```python
from build123d import *

# Parameters (mm, degrees)
SKETCH1_W            = 64.75
SKETCH1_H            = 20
BODY_DEPTH           = 140
SHELL1_T             = 3
SWITCH_CUTOUT_REACH  = 148.722
SKETCH2_W            = 26.75
SKETCH2_H            = 12
SKETCH4_W            = 15
SKETCH4_H            = 27
SKETCH4_R            = 4.0125
AXLE_HOLDER_DEPTH    = 15
SKETCH5_R            = 4.0125
SKETCH5_R_2          = 2.5
BUSHING_HOLDER_DEPTH = 9
FILLET3_R            = 4
FILLET4_R            = 6
SKETCH6_W            = 125
SKETCH6_H            = 10
SLIDE_MOUNT_DEPTH    = 3.5
CIRPATTERN1_COUNT    = 2
FILLET6_R            = 3
FILLET7_R            = 3
FILLET8_R            = 6
CUT_EXTRUDE1_REACH   = 147.177
SKETCH7_R            = 5.5
SKETCH8_R            = 8.916079783
CUT_EXTRUDE2_DEPTH   = 9
CUT_EXTRUDE3_DEPTH   = 3.5
CUT_EXTRUDE4_DEPTH   = 6.5


with BuildPart() as part:
    # Sketch1 → Body (new body)
    with BuildSketch(Plane.XY):
        Rectangle(SKETCH1_W, SKETCH1_H)
    extrude(amount=BODY_DEPTH)

    # Shell1
    shell1_openings = [part.faces().sort_by_distance(p)[0] for p in [
        (0, 0, 0),
        (0, 0, 140),
    ]]
    offset(amount=SHELL1_T, openings=shell1_openings, kind=Kind.INTERSECTION)

    # Sketch2 → Switch_cutout (cut, up to next)
    with BuildSketch(Plane(origin=(0, 13, 0), x_dir=(1, 0, 0), z_dir=(0, 1, 0)), mode=Mode.PRIVATE) as switch_cutout_sk1:
        with Locations((18, -6)):
            Rectangle(SKETCH2_W, SKETCH2_H)
    switch_cutout_tool1 = extrude(switch_cutout_sk1.sketch, amount=-SWITCH_CUTOUT_REACH, mode=Mode.PRIVATE) & part.part
    # Sketch2 → Switch_cutout (cut, up to next)
    with BuildSketch(Plane(origin=(0, 13, 0), x_dir=(1, 0, 0), z_dir=(0, 1, 0)), mode=Mode.PRIVATE) as switch_cutout_sk2:
        with Locations((-18, -134)):
            Rectangle(SKETCH2_W, SKETCH2_H)
    switch_cutout_tool2 = extrude(switch_cutout_sk2.sketch, amount=-SWITCH_CUTOUT_REACH, mode=Mode.PRIVATE) & part.part
    add(switch_cutout_tool1.solids().sort_by_distance((18, 13, 6))[0], mode=Mode.SUBTRACT)
    add(switch_cutout_tool2.solids().sort_by_distance((-18, 13, 134))[0], mode=Mode.SUBTRACT)

    # Sketch4 → Axle_holder (add, symmetric)
    # profile 1 of 2: a face of its own
    with BuildSketch(Plane.ZY):
        with Locations((12.5, -26.5)):
            Rectangle(SKETCH4_W, SKETCH4_H)
        with Locations(Location((12.5, -32.5, 0), (0, 0, 270))):
            Circle(SKETCH4_R, mode=Mode.SUBTRACT)
    # profile 2 of 2: a face of its own
    with BuildSketch(Plane.ZY):
        with Locations((127.5, -26.5)):
            Rectangle(SKETCH4_W, SKETCH4_H)
        with Locations(Location((127.5, -32.5, 0), (0, 0, 90))):
            Circle(SKETCH4_R, mode=Mode.SUBTRACT)
    extrude(amount=AXLE_HOLDER_DEPTH, both=True)

    # Sketch5 → Bushing_holder (add, symmetric)
    # profile 1 of 2: a face of its own
    with BuildSketch(Plane.ZY):
        with Locations(Location((12.5, -32.5, 0), (0, 0, 270))):
            Circle(SKETCH5_R)
        with Locations(Location((12.5, -32.5, 0), (0, 0, 270))):
            Circle(SKETCH5_R_2, mode=Mode.SUBTRACT)
    # profile 2 of 2: a face of its own
    with BuildSketch(Plane.ZY):
        with Locations(Location((127.5, -32.5, 0), (0, 0, 90))):
            Circle(SKETCH5_R)
        with Locations(Location((127.5, -32.5, 0), (0, 0, 270))):
            Circle(SKETCH5_R_2, mode=Mode.SUBTRACT)
    extrude(amount=BUSHING_HOLDER_DEPTH, both=True)

    # Fillet3
    fillet3_edges = [part.edges().sort_by_distance(p)[0] for p in [
        (0, -40, 5),
        (0, -40, 20),
        (0, -40, 135),
        (0, -40, 120),
    ]]
    fillet(fillet3_edges, radius=FILLET3_R)

    # Fillet4
    # the kernel refuses this fillet: 6 mm, written as the material it adds along each edge
    with BuildSketch(Plane(origin=(15, -13, 5), x_dir=(0, 0, -1), z_dir=(-1, 0, 0))) as fillet4_piece_1:
        with BuildLine():
            CenterArc((6, 5.916079783), FILLET4_R, 180, 80.405931773)
            Line((0, 5.916079783), (-0.12, 5.916079783))
            Line((-0.12, 5.916079783), (-0.12, 0))
            Line((-0.12, 0), (0, -0.12))
            ThreePointArc((0, -0.12), (2.5, -0.12), (4.98, -0.118321596))
            Line((4.98, -0.118321596), (5, 0))
        make_face()
    extrude(amount=30)
    with BuildSketch(Plane(origin=(-15, -13, 20), x_dir=(0, 0, 1), z_dir=(1, 0, 0)), Plane(origin=(-15, -13, 120), x_dir=(0, -1, 0), z_dir=(1, 0, 0))) as fillet4_piece_2:
        with BuildLine():
            CenterArc((FILLET4_R, FILLET4_R), FILLET4_R, 180, 90)
            Line((0, FILLET4_R), (-FILLET4_R * 0.02, FILLET4_R))
            Line((-FILLET4_R * 0.02, FILLET4_R), (-FILLET4_R * 0.02, -FILLET4_R * 0.02))
            Line((-FILLET4_R * 0.02, -FILLET4_R * 0.02), (FILLET4_R, -FILLET4_R * 0.02))
            Line((FILLET4_R, -FILLET4_R * 0.02), (FILLET4_R, 0))
        make_face()
    extrude(amount=30)
    with BuildSketch(Plane(origin=(15, -13, 135), x_dir=(0, 0, 1), z_dir=(-1, 0, 0))) as fillet4_piece_3:
        with BuildLine():
            CenterArc((6, -5.916079783), FILLET4_R, 99.594068227, 80.405931773)
            Line((0, -5.916079783), (-0.12, -5.916079783))
            Line((-0.12, -5.916079783), (-0.12, 0))
            Line((-0.12, 0), (0, 0.12))
            ThreePointArc((0, 0.12), (2.5, 0.12), (4.98, 0.118321596))
            Line((4.98, 0.118321596), (5, 0))
        make_face()
    extrude(amount=30)

    # Sketch6 → Slide_mount (add)
    with BuildSketch(Plane(origin=(35.375, 0, 0), x_dir=(0, 0, -1), z_dir=(1, 0, 0))):
        with Locations((-77.5, 18)):
            Rectangle(SKETCH6_W, SKETCH6_H)
        with BuildLine():
            Line((-132, 18.7), (-23, 18.7))
            ThreePointArc((-23, 18.7), (-21.3, 17), (-23, 15.3))
            Line((-23, 15.3), (-132, 15.3))
            ThreePointArc((-132, 15.3), (-133.7, 17), (-132, 18.7))
        make_face(mode=Mode.SUBTRACT)
    slide_mount = extrude(amount=-SLIDE_MOUNT_DEPTH)

    # CirPattern1: Slide_mount ×2 about axis
    cirpattern1_axis = Axis((0, 0, 70), (0, 1, 0))
    for i in range(1, CIRPATTERN1_COUNT):
        add(slide_mount.rotate(cirpattern1_axis, i * 360 / CIRPATTERN1_COUNT))

    # Fillet6
    fillet6_edges = [part.edges().sort_by_distance(p)[0] for p in [
        (33.625, 23, 140),
        (33.625, 23, 15),
        (-33.625, 23, 0),
        (-33.625, 23, 125),
    ]]
    fillet(fillet6_edges, radius=FILLET6_R)

    # Fillet7
    fillet7_edges = [part.edges().sort_by_distance(p)[0] for p in [
        (4.625, 11.5, 12),
        (31.375, 11.5, 12),
        (-31.375, 11.5, 128),
        (-4.625, 11.5, 128),
    ]]
    fillet(fillet7_edges, radius=FILLET7_R)

    # Fillet8
    fillet8_edges = [part.edges().sort_by_distance(p)[0] for p in [
        (33.625, 13, 15),
        (-33.625, 13, 125),
    ]]
    fillet(fillet8_edges, radius=FILLET8_R)

    # Sketch7 → Cut-Extrude1 (cut, up to next)
    with BuildSketch(Plane.XY.offset(135), mode=Mode.PRIVATE) as cut_extrude1_sk1:
        with Locations(Location((0, -21.916079783, 0), (0, 0, 32.018720622))):
            Circle(SKETCH7_R)
    cut_extrude1_tool1 = extrude(cut_extrude1_sk1.sketch, amount=-CUT_EXTRUDE1_REACH, mode=Mode.PRIVATE) & part.part
    add(cut_extrude1_tool1.solids().sort_by_distance((0, -21.91608, 135))[0], mode=Mode.SUBTRACT)

    # Sketch8 → Cut-Extrude2 (cut)
    with BuildSketch(Plane.XY.offset(135)):
        with Locations((0, -21.916079783)):
            Circle(SKETCH8_R)
    extrude(amount=CUT_EXTRUDE2_DEPTH, mode=Mode.SUBTRACT)

    # Sketch9 → Cut-Extrude3 (cut, symmetric)
    with BuildSketch(Plane(origin=(0, 0, 120), x_dir=(-1, 0, 0), z_dir=(0, 0, -1))):
        Polygon((-9.814954576, -21.916079783), (-4.907477288, -30.416079783), (4.907477288, -30.416079783), (9.814954576, -21.916079783), (4.907477288, -13.416079783), (-4.907477288, -13.416079783), align=None)
    extrude(amount=CUT_EXTRUDE3_DEPTH, both=True, mode=Mode.SUBTRACT)

    # Sketch10 → Cut-Extrude4 (cut)
    with BuildSketch(Plane.XY.offset(135)):
        Polygon((3.464101615, -15.916079783), (-3.464101615, -15.916079783), (-6.92820323, -21.916079783), (-3.464101615, -27.916079783), (3.464101615, -27.916079783), (6.92820323, -21.916079783), align=None)
    extrude(amount=-CUT_EXTRUDE4_DEPTH, mode=Mode.SUBTRACT)


solid = part.part
```
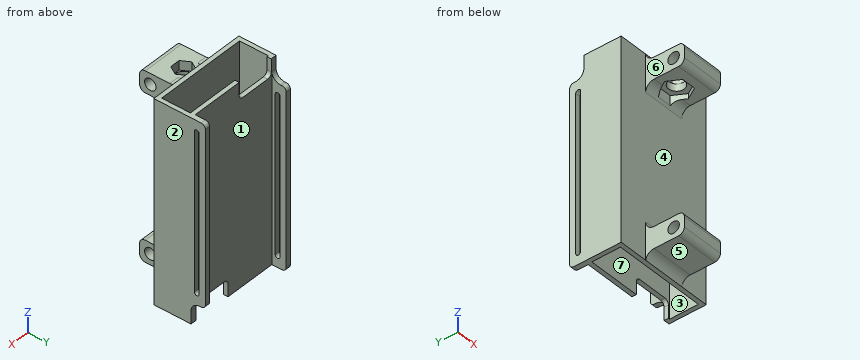
Build history of the part. All positions in model axes, mm. Face numbers are marked on the shaded views. A direction names the side the tool comes from. Coordinates: 2 decimals unless noted, no trailing zeros. Order: outer loops, then holes, each group sorted by start corner. A loop starts at its lowest first (then second) coordinate and runs counter-clockwise, first axis right, second up.
Item 1: Saw through at A-A on x = 13. List the corners of the cut face in (y, z) (1 decimal), then the cut area to 3 significant figures.
Filled in:
outline: (-40, 9) arc R4 ccw to (-36, 5) - (-18.9, 5) arc R6 cw to (-13, 0) - (-10, 0) - (-10, 140) - (-13, 140) arc R6 cw to (-18.9, 135) - (-36, 135) arc R4 ccw to (-40, 131) - (-40, 124) arc R4 ccw to (-36, 120) - (-19, 120) arc R6 cw to (-13, 114) - (-13, 26) arc R6 cw to (-19, 20) - (-36, 20) arc R4 ccw to (-40, 16) - close; (10, 12) - (13, 12) - (13, 140) - (10, 140) - close; hole circle Ø8 at (-32.5, 12.5); hole circle Ø8 at (-32.5, 127.5)
area: 1,530 mm2
Item 2: Saw through at C-C on y = -6.5. List the corners of the cut face in (x, z) (3 decimals).
Filled in:
outline: (-35.375, 0) - (-32.375, 0) - (-32.375, 140) - (-35.375, 140) - close; (32.375, 0) - (35.375, 0) - (35.375, 140) - (32.375, 140) - close
Item 3: Drop flat-ended pins along their axis: pin 1 Ø0.5 at (x, y) = (-34, 19.5) entering from +Z; pin 2 Ø5 at (x, z) = (-11.5, 113) entering from +Y; pin 3 Ø10.5 at (y, z) = (-32.5, 12.5) entering from +X; pin 4 Ø5 at (y, z) = (18, 82.5) entering from -X (3 decimals). Give the stop position or say it passes through.
Filled in:
pin 1: stops at z = 125
pin 2: stops at y = 13
pin 3: stops at x = 15
pin 4: stops at x = -35.375
Item 4: Mould opens along Y. For the marked faces 1, 2 and 3 say: released by +Y, released by -Y, zero draft, split by the parting line, or undercut.
Filled in:
face 1: released by +Y
face 2: zero draft
face 3: undercut
Item 5: Drill centre lines: L1, parallel to Y at x = 12.05, z = 127.5; L2, parallel to Z at x = 10.6, y = -32.5; L3, parallel to Z at x = 3.75, y = -32.5. Where is each one in solid material? Low to high.
Filled in:
L1: y = -40 to -36.51, -28.49 to -10, 10 to 13
L2: z = 5 to 8.49, 16.51 to 20, 120 to 123.49, 131.51 to 135
L3: z = 5 to 10, 15 to 20, 120 to 125, 130 to 135
Item 6: Saw through at B-B on z = 33. List the corners of the cut face in (x, y) (3 decimals).
Filled in:
outline: (-35.375, -13) - (35.375, -13) - (35.375, 15.3) - (31.875, 15.3) - (31.875, 13) - (-31.875, 13) - (-31.875, 15.3) - (-35.375, 15.3) - close; (-35.375, 18.7) - (-31.875, 18.7) - (-31.875, 23) - (-35.375, 23) - close; (31.875, 18.7) - (35.375, 18.7) - (35.375, 23) - (31.875, 23) - close; hole (-32.375, -10) - (32.375, -10) - (32.375, 10) - (-32.375, 10) - close
Item 7: Tool access for the marked faces 4, 5, 6 and 7: list every direction of +Z, -Z, +X, -X, +Y, -Y with a clear straight run to the whole face (end or side of a thin tool).
Filled in:
face 4: -Y
face 5: -Z, +X, -X, -Y
face 6: +Z, -Z, -X, -Y
face 7: +Z, -Z
Item 8: Saw through at D-D on y = 17. List the corners of the cut face in (x, z) (3 decimals).
Filled in:
outline: (-35.375, 0) - (-31.875, 0) - (-31.875, 6.3) - (-35.375, 6.3) - close; (-35.375, 118.7) - (-31.875, 118.7) - (-31.875, 125.343) - (-35.375, 125.343) - close; (31.875, 14.657) - (35.375, 14.657) - (35.375, 21.3) - (31.875, 21.3) - close; (31.875, 133.7) - (35.375, 133.7) - (35.375, 140) - (31.875, 140) - close
